Print and shaded views of the part. All mm, measured from the part's lowest x, y and z. A direction names the side the tool comes from. Round coordinates to 2 decimals unless told otherwise and drop trailing zeros. Write each loop counter-clockwise with the first axis right and the second up, starting at its lowest first coordinate (ties: lowest second). Pieces come first, ordered by that corner, then holes.
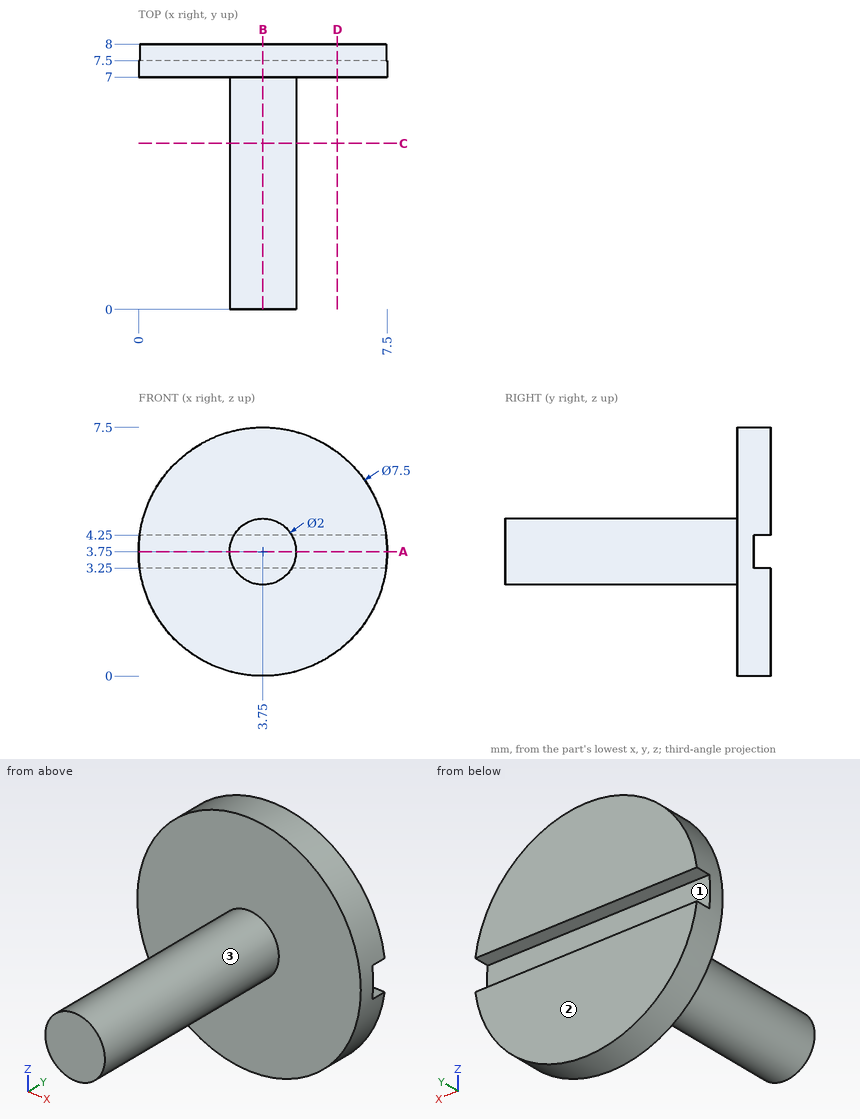
1) Slice it at B-B (x = 3.75). Write the cut outline in (y, z), plus the area to 3 significant figures.
Results:
outline: (0, 2.75) - (7, 2.75) - (7, 0) - (8, 0) - (8, 3.25) - (7.5, 3.25) - (7.5, 4.25) - (8, 4.25) - (8, 7.5) - (7, 7.5) - (7, 4.75) - (0, 4.75) - close
area: 21.0 mm2
2) Slice it at A-A (z = 3.75). Write the cut outline in (x, y), plus the area to 4 significant figures.
Results:
outline: (0, 7) - (2.75, 7) - (2.75, 0) - (4.75, 0) - (4.75, 7) - (7.5, 7) - (7.5, 7.5) - (0, 7.5) - close
area: 17.75 mm2
3) Slice it at C-C (y = 5). Write the cut outline in (x, z), plus the area to 3 significant figures.
Results:
outline: circle Ø2 at (3.75, 3.75)
area: 3.14 mm2
4) Pin check, flat tips, straight feed: pin 1 Ø1.5 at (x, z) = (1, 2) entering from -Y; pin 2 Ø3 at (y, z) = (3, 6) entering from -X; pin 3 Ø3 at (y, z) = (3.5, 3.5) entering from -X; pin 4 Ø1 at (y, z) = (5.5, 6.5) entering from +X. Stop position of each tip, or through.
Results:
pin 1: stops at y = 7
pin 2: stops at x = 3.09
pin 3: stops at x = 2.75
pin 4: passes through
5) Slice it at D-D (x = 6). Write the cut outline in (y, z), plus the area to 3 significant figures.
Results:
outline: (7, 0.75) - (8, 0.75) - (8, 3.25) - (7.5, 3.25) - (7.5, 4.25) - (8, 4.25) - (8, 6.75) - (7, 6.75) - close
area: 5.50 mm2
6) Wall check: L1, parallel to Y at x = 6.75, z = 1.75; L2, parallel to Y at x = 1, z = 3.5; L3, parallel to Z at x = 3, y = 6.5. Give the ranges that are in metal, low to high.
Results:
L1: y = 7 to 8
L2: y = 7 to 7.5
L3: z = 3.09 to 4.41
7) Which spindle directions (+Z, -Z, +X, -X, +Y, -Y) get a long thin tool onto all of the face, cutting with end or side? Do the marked faces 1, 2 and 3. Say none if no direction does.
Results:
face 1: +X, -X, +Y
face 2: +Z, -Z, +X, -X, +Y
face 3: -Y
